Source: CAD feature listing. Evaluate the final solid. Frame: model axes, mm. A direction names the side the tool comes from. Round coordinates to 2 decimals unless told otherwise and drop trailing zeros. Order: outer loops, then holes, each group sorted by start corner. A loop starts at its lowest first (then second) coordinate and runs counter-clockwise, first axis right, second up. Notation, with made-up numbers: M 27,59 L 39,59 A18 ccw 39,63 Z; hole C -3,-3.5 d3. An arc over 180 degrees is marked long. Use CSV: the item, a comma, the result in double quotes. Start each with the question number.
```python
from build123d import *

# Parameters (mm, degrees)
CROQUIS1_R              = 11.5
CROQUIS1_R_2            = 1.6
SALIENTE_EXTRUIR1_DEPTH = 3
CROQUIS2_W              = 10
CROQUIS2_H              = 10
CROQUIS2_R              = 2.15
SALIENTE_EXTRUIR2_DEPTH = 7


with BuildPart() as part:
    # Croquis1 → Saliente-Extruir1 (new body)
    with BuildSketch(Plane.XY):
        Polygon((21.15, 17.15), (17.15, 21.15), (-17.15, 21.15), (-21.15, 17.15), (-21.15, -17.15), (-17.15, -21.15), (17.15, -21.15), (21.15, -17.15), align=None)
        Circle(CROQUIS1_R, mode=Mode.SUBTRACT)
        with Locations((15.5, 15.5)):
            Circle(CROQUIS1_R_2, mode=Mode.SUBTRACT)
        with Locations((15.5, -15.5)):
            Circle(CROQUIS1_R_2, mode=Mode.SUBTRACT)
        with Locations((-15.5, -15.5)):
            Circle(CROQUIS1_R_2, mode=Mode.SUBTRACT)
        with Locations((-15.5, 15.5)):
            Circle(CROQUIS1_R_2, mode=Mode.SUBTRACT)
    extrude(amount=SALIENTE_EXTRUIR1_DEPTH)

    # Croquis2 → Saliente-Extruir2 (add)
    with BuildSketch(Plane(origin=(21.15, 0, 0), x_dir=(0, 0, -1), z_dir=(1, 0, 0))):
        with Locations((-8, 6.15)):
            Rectangle(CROQUIS2_W, CROQUIS2_H)
        with Locations((-8, 6.15)):
            Circle(CROQUIS2_R, mode=Mode.SUBTRACT)
    extrude(amount=-SALIENTE_EXTRUIR2_DEPTH)


solid = part.part
```
(1) Line query: line 1 along Y through (x, z) = (-15.5, 1.95); line 2 along Y through (x, z) = (0, 1.6); line 3 along X through (y, z) = (9, 4). Output: solid intervals per line, ascending.
(2) Reachability of faces 1 (the face through (14.15, 6.2, 10.3)), 2 (the face through (17.699, 5.327, 6.014)), 3 (the face through (18, 1.15, 8)) from +Z, -Z, +X, -X, +Y, -Y: full face, straight path, thin tool, end or side. Return the list, or none.
(3) Section B-B on y = 0. Return loops of the section in (x, z), plus the area to 3 significant figures.
(4) Section D-D on z = 8. Return loops of the section in (x, y).
(5) Draft query along Y for faces 4 (the face through (21.15, 2, 5)), 5 (the face through (-1.5, 11.4, 1.5)), 6 (the face through (19.1, -19.2, 1.5)). Return one class per face: pulls with the +Y half, pulls with the -Y half, needs draft (parallel to the pull), parting line crosses it, or undercut.
(6) Section C-C on y = 15.5. Return loops of the section in (x, z).
(7) Section A-A on x = 15.5. Return loops of the section in (y, z), plus the area to 3 significant figures.
(8) Contact query for flat-ended pins moving along their axis: P1, Ø4, axis at x = -15.5, y = 15.5, coming from the +Z side; P2, Ø2, axis at x = 17.5, z = 7, coming from the -Y side; P3, Ø1, axis at y = -8.5, z = 4, coming from the +X side; P4, Ø5, axis at y = 4, z = 6.5, coming from the -X side. Output: stop coordinate, or through.
Results below:
1,line 1,"y = -21.15 to -17.1, -13.9 to 13.9, 17.1 to 21.15"
1,line 2,"y = -21.15 to -11.5, 11.5 to 21.15"
1,line 3,"x = 14.15 to 21.15"
2,face 1,"+Z, -X, +Y, -Y"
2,face 2,"+X, -X"
2,face 3,"+Z, +X, -X, -Y"
3,outline,"M -21.15,0 L -11.5,0 L -11.5,3 L -21.15,3 Z; M 11.5,0 L 21.15,0 L 21.15,3 L 11.5,3 Z"
3,area,"57.9 mm2"
4,outline,"M 14.15,1.15 L 21.15,1.15 L 21.15,4 L 14.15,4 Z; M 14.15,8.3 L 21.15,8.3 L 21.15,11.15 L 14.15,11.15 Z"
5,face 4,"needs draft"
5,face 5,"undercut"
5,face 6,"pulls with the -Y half"
6,outline,"M -21.15,0 L -17.1,0 L -17.1,3 L -21.15,3 Z; M -13.9,0 L 13.9,0 L 13.9,3 L -13.9,3 Z; M 17.1,0 L 21.15,0 L 21.15,3 L 17.1,3 Z"
7,outline,"M -21.15,0 L -17.1,0 L -17.1,3 L -21.15,3 Z; M -13.9,0 L 13.9,0 L 13.9,3 L 11.15,3 L 11.15,13 L 1.15,13 L 1.15,3 L -13.9,3 Z; M 17.1,0 L 21.15,0 L 21.15,3 L 17.1,3 Z; hole C 6.15,8 d4.3"
7,area,"193 mm2"
8,P1,"stops at z = 3"
8,P2,"stops at y = 1.15"
8,P3,"passes through"
8,P4,"stops at x = 14.15"
